Here's how the part is built. I have some questions about the finished solid (model axes, mm). A direction names the side the tool comes from. Give positions to 0.01 mm unless a question says otherwise; leave off trailing zeros. Write each loop counter-clockwise with the first axis right and the second up, starting at its lowest first coordinate (ties: lowest second). Pieces come first, ordered by that corner, then holes. Notation, with made-up numbers: (66.5, 66) - (90.5, 66) arc R11 ccw to (90.5, 70) - close; hole circle Ø5 at (66, -9). An arc over 180 degrees is marked (long way). Use a Markdown table: item, result.
```python
from build123d import *

# Parameters (mm, degrees)
SKETCH1_R               = 30
BOSS_EXTRUDE1_DEPTH     = 330
CUT_EXTRUDE1_DEPTH      = 333.716095192
CUT_EXTRUDE1_DEPTH_BACK = 333.716095192
SKETCH2_R               = 10.05
CUT_EXTRUDE2_DEPTH      = 335.89140043
SKETCH4_OUTSIDE_W       = 195.086
SKETCH4_OUTSIDE_H       = 195.086
SKETCH4_OUTSIDE_W_2     = 46
SKETCH4_OUTSIDE_H_2     = 46
CUT_EXTRUDE3_DEPTH      = 30
SKETCH5_OUTSIDE_W       = 195.086
SKETCH5_OUTSIDE_H       = 195.086
SKETCH5_OUTSIDE_R       = 24.61
CUT_EXTRUDE4_DEPTH      = 200
SKETCH6_OUTSIDE_W       = 195.086
SKETCH6_OUTSIDE_H       = 195.086
SKETCH6_OUTSIDE_R       = 25
CUT_EXTRUDE5_DEPTH      = 430


with BuildPart() as part:
    # Sketch1 → Boss-Extrude1 (new, symmetric)
    with BuildSketch(Plane.XY):
        Circle(SKETCH1_R)
    extrude(amount=BOSS_EXTRUDE1_DEPTH, both=True)

    # Sketch2 → Cut-Extrude1 (cut, two sides: drawn at the far end of the back side and taken through both)
    with BuildSketch(Plane(origin=(0, 0, 0), x_dir=(0, 0, -1), z_dir=(1, 0, 0)).offset(-CUT_EXTRUDE1_DEPTH_BACK)):
        with Locations(Location((190, 0, 0), (0, 0, 180))):
            Circle(SKETCH2_R)
        with Locations(Location((290, 0, 0), (0, 0, 180))):
            Circle(SKETCH2_R)
    extrude(amount=CUT_EXTRUDE1_DEPTH + CUT_EXTRUDE1_DEPTH_BACK, mode=Mode.SUBTRACT)

    # Sketch3 → Cut-Extrude2 (cut, through all)
    with BuildSketch(Plane(origin=(-18.5, 0, 0), x_dir=(0, 0, -1), z_dir=(1, 0, 0))):
        with BuildLine():
            Line((-215, -7), (-173, -7))
            ThreePointArc((-173, -7), (-166, 0), (-173, 7))
            Line((-173, 7), (-215, 7))
            ThreePointArc((-215, 7), (-222, 0), (-215, -7))
        make_face()
    extrude(amount=-CUT_EXTRUDE2_DEPTH, mode=Mode.SUBTRACT)

    # Sketch4 outside → Cut-Extrude3 (cut)
    with BuildSketch(Plane.XY.offset(330)):
        Rectangle(SKETCH4_OUTSIDE_W, SKETCH4_OUTSIDE_H)
        Rectangle(SKETCH4_OUTSIDE_W_2, SKETCH4_OUTSIDE_H_2, mode=Mode.SUBTRACT)
    extrude(amount=-CUT_EXTRUDE3_DEPTH, mode=Mode.SUBTRACT)

    # Sketch5 outside → Cut-Extrude4 (cut)
    with BuildSketch(Plane(origin=(0, 0, -330), x_dir=(-1, 0, 0), z_dir=(0, 0, -1))):
        Rectangle(SKETCH5_OUTSIDE_W, SKETCH5_OUTSIDE_H)
        Circle(SKETCH5_OUTSIDE_R, mode=Mode.SUBTRACT)
    extrude(amount=-CUT_EXTRUDE4_DEPTH, mode=Mode.SUBTRACT)

    # Sketch6 outside → Cut-Extrude5 (cut)
    with BuildSketch(Plane(origin=(0, 0, -130), x_dir=(-1, 0, 0), z_dir=(0, 0, -1))):
        Rectangle(SKETCH6_OUTSIDE_W, SKETCH6_OUTSIDE_H)
        Circle(SKETCH6_OUTSIDE_R, mode=Mode.SUBTRACT)
    extrude(amount=-CUT_EXTRUDE5_DEPTH, mode=Mode.SUBTRACT)


solid = part.part
```
Item 1: I need wall thicknesses on line 1 along Z through (x, y) = (17, 1.5); line 2 along Y through (x, z) = (0, -190); line 3 along Z through (x, y) = (22, -19). Which ranges of each line are inside material? Lowest first, please. Write a range as [from, to].
Values:
| item | result |
|---|---|
| line 1 | z = [-330, -299.94], [-280.06, -199.94], [-180.06, 330] |
| line 2 | y = [-24.61, -10.05], [10.05, 24.61] |
| line 3 | z = [300, 330] |
Item 2: For faces 5 (the flat face through (0, -23, 315)), 6 (the flat face through (-19, 19, 300)), 7 (the cylindrical face through (-23.846, 7.509, 81.99)), which set-ups out of +Z, -Z, +X, -X, +Y, -Y let a thin tool reach every point of the face, with its end or its side?
Values:
| item | result |
|---|---|
| face 5 | +Z, +X, -X, -Y |
| face 6 | -Z, -X, +Y |
| face 7 | -Z |
Item 3: If we section it at C-C, the plane z = -290: Write out the boundary of the cut face in (x, y), plus the area to 3 significant figures.
Values:
| item | result |
|---|---|
| outline | (-22.46, -10.05) arc R24.61 ccw to (22.46, -10.05) - close; (-22.46, 10.05) - (22.46, 10.05) arc R24.61 ccw to start |
| area | 942 mm2 |
Item 4: If we section it at A-A, the plane x = -2.5: Write out the boundary of the cut face in (y, z).
Values:
| item | result |
|---|---|
| outline | (-24.87, -130) - (-24.48, -130) - (-24.48, -330) - (24.48, -330) - (24.48, -130) - (24.87, -130) - (24.87, 300) - (23, 300) - (23, 330) - (-23, 330) - (-23, 300) - (-24.87, 300) - close; hole circle Ø20.1 at (0, -290); hole circle Ø20.1 at (0, -190) |
Item 5: If we section it at D-D, the plane z = -191: Write out the boundary of the cut face in (x, y).
Values:
| item | result |
|---|---|
| outline | (-22.49, -10) arc R24.61 ccw to (22.49, -10) - close; (-22.49, 10) - (22.49, 10) arc R24.61 ccw to start |
Item 6: Thinking about a two-plate mould opening in Z: for faces 1 (the flat face through (-23, 0, 315)), 2 (the flat face through (19, 18, 300)), 3 (the flat face through (0, 0, 330)), 4 (the flat face through (-18.5, 0, 194)), which applies, +Z half, -Z half, draft (parallel to the pull), parting line (faces both ways), or undercut?
Values:
| item | result |
|---|---|
| face 1 | draft |
| face 2 | -Z half |
| face 3 | +Z half |
| face 4 | undercut |
Item 7: Will these pins go through, and if not, where does the flat tip stop? pin 1 Ø3 at (y, z) = (18.5, -88) entering from +X; pin 2 Ø11 at (y, z) = (-1, 197) entering from -X; pin 3 Ø0.6 at (x, y) = (-4, -23.5) entering from +Z; pin 4 Ø8 at (y, z) = (3.5, 176.5) entering from +X.
Values:
| item | result |
|---|---|
| pin 1 | stops at x = 18.33 |
| pin 2 | stops at x = -18.5 |
| pin 3 | stops at z = 300 |
| pin 4 | stops at x = 25 |
Item 8: If we section it at B-B, the plane z = 111.5: Write out the boundary of the cut face in (x, y), plus the area to 3 significant figures.
Values:
| item | result |
|---|---|
| outline | circle Ø50 at (0, 0) |
| area | 1,960 mm2 |
